Can you work these out from the model? Positions are in its coordinate system, mm. Face numbers are marked on the shaded views. Round coordinates to 2 decimals unless told otherwise and drop trailing zeros. Order: outer loops, then holes, each group sorted by start corner. A loop starts at its lowest first (then second) coordinate and runs counter-clockwise, first axis right, second up. Notation, with made-up numbers: (27.5, 4.25) -> (53.5, 4.25) arc R25 cw to (53.5, 34.25) -> close; hole circle Ø6 at (6.5, 34). An arc over 180 degrees is marked (long way). Use a Markdown table: item, result. Add a question column.
Q1. If we section it at B-B on x = 147: List the corners of the cut face in (y, z) for me, plus the area to 4 significant figures.
Q2. I'm going to push flat-ended pins straight in: pin 1 Ø4 at (x, y) = (99, 4) entering from +Z; pin 2 Ø3 at (x, y) = (148, 5) entering from +Z; pin 3 Ø3 at (y, z) = (5, 11.5) entering from -X. Where does each tip first touch, or does it pass through?
Q3. If we section it at C-C on x = 15: List the corners of the cut face in (y, z) for me.
Q4. If we section it at A-A on x = 88.5: List the corners of the cut face in (y, z) for me, plus the area to 3 significant figures.
Q5. We'd pull the mould along X, two halves only. Please class the marked faces 1 and 2: +X half, -X half, draft (parallel to the pull), parting line (faces both ways), or undercut.
Q6. I need wall thicknesses on line 1 along Y through (x, z) = (15, 1.55); line 2 along Z through (x, y) = (125, 3); line 3 along Z through (x, y) = (150, 6.25). Which ranges of each line are inside material? Lowest first, please. Write a range as [from, to].
Autodesk Inventor part; units mm, degrees
ref_plane "YZ Plane" through (0, 0, 0) normal (1, 0, 0) x (0, 1, 0)
ref_plane "XZ Plane" through (0, 0, 0) normal (0, 1, 0) x (-1, 0, 0)
ref_plane "XY Plane" through (0, 0, 0) normal (0, 0, 1) x (1, 0, 0)
sketch "Sketch1" plane through (0, 0, 0) normal (0, 0, 1) x (1, 0, 0)
  line L0 (0, 0) -> (164.5, 0)
  line L1 (164.5, 0) -> (164.5, 9)
  line L2 (164.5, 9) -> (0, 9)
  line L3 (0, 9) -> (0, 0)
  circle A0 centre (57, 4) radius 1.6
  circle A1 centre (99, 4) radius 1.6
  circle A2 centre (159.5, 4) radius 1.6
  circle A3 centre (147, 4) radius 1.6
  circle A4 centre (15, 4) radius 1.6
  circle A5 centre (7, 4) radius 1.6
  dimension "d1" = 9
  dimension "d2" = 90
  dimension "d4" = 3.2
  dimension "d6" = 3.2
  dimension "d7" = 3.2
  dimension "d8" = 42
  dimension "d9" = 60.5
  dimension "d26" = 3.2
  dimension "d27" = 48
  dimension "d28" = 3.2
  dimension "d29" = 42
  dimension "d32" = 15
  dimension "d33" = 5
  dimension "d61" = 3.2
  dimension "d62" = 8
  dimension "d63" = 12.5
  dimension "d108" = 4
  dimension "d109" = 4
  dimension "d110" = 4
  dimension "d111" = 4
  dimension "d112" = 4
  dimension "d113" = 4
ref_plane "Work Plane2" through (0, 0, 0) normal (0, -1, 0) x (1, 0, 0)
sketch "Sketch2" plane through (0, 0, 0) normal (0, -1, 0) x (1, 0, 0)
  circle A0 centre (52, 10) radius 1.6
  circle A1 centre (125, 10) radius 1.6
  circle A2 centre (88.5, 10) radius 1.6
  point P0 (0, 0)
  point P1 (52, 0)
  dimension "d13" = 3.2
  dimension "d15" = 3.2
  dimension "d17" = 3.2
  dimension "d18" = 36.5
  dimension "d64" = 52
  dimension "d65" = 36.5
  dimension "d114" = 10
  dimension "d115" = 73
ref_plane "Work Plane1" through (0, 0, 11) normal (0, 0, 1) x (1, 0, 0)
extrude "klocek" add sketch "Sketch1" along normal blind 13
ref_plane "Work Plane3" through (0, 0, 0) normal (0, -1, 0) x (1, 0, 0)
extrude "prowadzenie osi" cut sketch "Sketch2" against normal up to next
ref_plane "Work Plane4" through (0, 0, 0) normal (0, -1, 0) x (1, 0, 0)
sketch "Sketch7" plane through (0, 0, 0) normal (0, -1, 0) x (1, 0, 0)
  line L0 (0, 13) -> (0, 1)
  line L1 (0, 13) -> (164.5, 13)
  line L2 (0, 13) -> (40, 13)
  line L3 (40, 13) -> (0, 1)
  point P0 (0, -1.8333)
  dimension "d86" = 12
  dimension "d87" = 40
sketch "Sketch8" plane through (0, 0, 0) normal (0, -1, 0) x (1, 0, 0)
  line L0 (164.5, 0) -> (164.5, 13)
  line L1 (164.5, 13) -> (164.5, 1)
  line L2 (164.5, 13) -> (0, 13)
  line L3 (164.5, 13) -> (134.5, 13)
  line L4 (134.5, 13) -> (164.5, 1)
  point P0 (0, 0)
  point P1 (40.8333, 11)
  dimension "d80" = 12
  dimension "d81" = 30
extrude "przedni skos" cut sketch "Sketch7" against normal up to next
extrude "tylni skos" cut sketch "Sketch8" against normal up to next
ref_plane "Work Plane7" through (0, 0, 11) normal (0, 0, 1) x (1, 0, 0)
sketch "Sketch5" plane through (0, 0, 13) normal (0, 0, 1) x (1, 0, 0)
  circle A0 centre (99, 4) radius 1.6
  line L0 (95.5936, 4) -> (97.2968, 6.95)
  line L1 (97.2968, 6.95) -> (100.7032, 6.95)
  line L2 (100.7032, 6.95) -> (102.4064, 4)
  line L3 (102.4064, 4) -> (100.7032, 1.05)
  line L4 (100.7032, 1.05) -> (97.2968, 1.05)
  line L5 (97.2968, 1.05) -> (95.5936, 4)
  circle A1 centre (57, 4) radius 1.6
  line L6 (60.4064, 4) -> (58.7032, 1.05)
  line L7 (58.7032, 1.05) -> (55.2968, 1.05)
  line L8 (55.2968, 1.05) -> (53.5936, 4)
  line L9 (53.5936, 4) -> (55.2968, 6.95)
  line L10 (55.2968, 6.95) -> (58.7032, 6.95)
  line L11 (58.7032, 6.95) -> (60.4064, 4)
  point P0 (119.5, 5)
  dimension "d98" = 5.9
  dimension "d100" = 5.9
extrude "hex insert middle" cut sketch "Sketch5" against normal blind 3
ref_plane "Work Plane6" through (0, 0, 11) normal (0, 0, 1) x (1, 0, 0)
sketch "Sketch9" plane through (0, 0, 11) normal (0, 0, 1) x (1, 0, 0)
  circle A0 centre (147, 4) radius 1.6
  line L0 (150.4064, 4) -> (148.7032, 1.05)
  line L1 (148.7032, 1.05) -> (145.2968, 1.05)
  line L2 (145.2968, 1.05) -> (143.5936, 4)
  line L3 (143.5936, 4) -> (145.2968, 6.95)
  line L4 (145.2968, 6.95) -> (148.7032, 6.95)
  line L5 (148.7032, 6.95) -> (150.4064, 4)
  point P0 (0, 0)
  point P1 (153, 5)
  dimension "d99" = 5.9
extrude "hex insert rear 1" cut sketch "Sketch9" against normal blind 7.5
ref_plane "Work Plane5" through (0, 0, 11) normal (0, 0, 1) x (1, 0, 0)
sketch "Sketch10" plane through (0, 0, 11) normal (0, 0, 1) x (1, 0, 0)
  circle A0 centre (159.5, 4) radius 1.6
  line L0 (162.45, 5.7032) -> (162.45, 2.2968)
  line L1 (162.45, 2.2968) -> (159.5, 0.5936)
  line L2 (159.5, 0.5936) -> (156.55, 2.2968)
  line L3 (156.55, 2.2968) -> (156.55, 5.7032)
  line L4 (156.55, 5.7032) -> (159.5, 7.4064)
  line L5 (159.5, 7.4064) -> (162.45, 5.7032)
  line L6 (164.5, 0) -> (134.5, 0)
  point P0 (0, 0)
  dimension "d118" = 5.9
extrude "hex insert rear 2" cut sketch "Sketch10" against normal up to next contours A0 | L0 L1 L2 L3 L4 L5
sketch "Sketch13" plane through (0, 0, 11) normal (0, 0, 1) x (1, 0, 0)
  circle A0 centre (7, 4) radius 1.6
  line L0 (10.4064, 4) -> (8.7032, 1.05)
  line L1 (8.7032, 1.05) -> (5.2968, 1.05)
  line L2 (5.2968, 1.05) -> (3.5936, 4)
  line L3 (3.5936, 4) -> (5.2968, 6.95)
  line L4 (5.2968, 6.95) -> (8.7032, 6.95)
  line L5 (8.7032, 6.95) -> (10.4064, 4)
  dimension "d123" = 5.9
extrude "hex insert front 1" cut sketch "Sketch13" against normal through all
sketch "Sketch16" plane through (0, 0, 11) normal (0, 0, 1) x (1, 0, 0)
  circle A0 centre (15, 4) radius 1.6
  line L0 (18.4064, 4) -> (16.7032, 1.05)
  line L1 (16.7032, 1.05) -> (13.2968, 1.05)
  line L2 (13.2968, 1.05) -> (11.5936, 4)
  line L3 (11.5936, 4) -> (13.2968, 6.95)
  line L4 (13.2968, 6.95) -> (16.7032, 6.95)
  line L5 (16.7032, 6.95) -> (18.4064, 4)
  point P0 (0, 0)
  dimension "d93" = 5.9
extrude "hex insert front 2" cut sketch "Sketch16" against normal blind 9
sketch "Sketch17" plane through (0, 0, 0) normal (0, 0, -1) x (-1, 0, 0)
  line L0 (-164.5, 9) -> (0, 9)
  line L1 (0, 0) -> (-2, 0)
  line L2 (-2, 0) -> (-2, 9)
  line L3 (-2, 9) -> (0, 9)
  line L4 (0, 9) -> (0, 0)
  dimension "d122" = 2
extrude "ciecie przod" cut sketch "Sketch17" against normal up to next
sketch "Sketch18" plane through (40, 0, 13) normal (0, -1, 0) x (1, 0, 0)
  line L0 (9.5, 0) -> (9.5, -4)
  line L1 (9.5, -4) -> (-15.5, -4)
  line L2 (-15.5, -4) -> (-15.5, 0)
  line L3 (-15.5, 0) -> (9.5, 0)
  line L4 (94.5, 0) -> (0, 0)
  circle A0 centre (12, -3) radius 1.6
  line L5 (-40, -13) -> (124.5, -13)
  point P0 (-35, -11)
  dimension "d102" = 4
  dimension "d103" = 25
  dimension "d104" = 2.5
extrude "sensor linii" cut sketch "Sketch18" against normal blind 7.3 contours L0 L1 L2 L3
properties part number "wheel_support_v5_narrow_with_line_sensor_all_holes_2mm_higher"
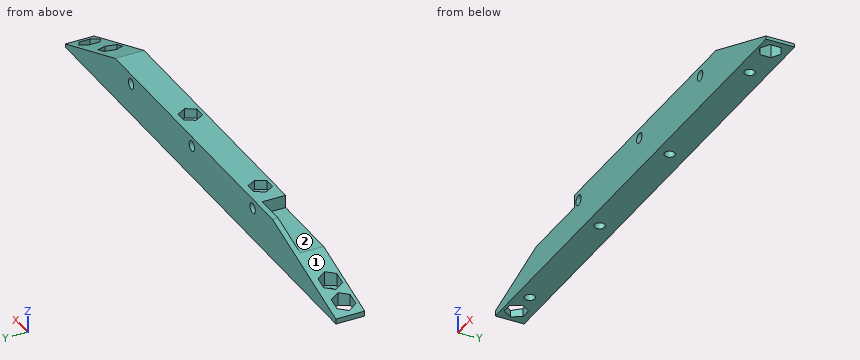
Answer below:
| question | item | result |
|---|---|---|
| 1 | outline | (0, 0) -> (2.4, 0) -> (2.4, 3.5) -> (1.05, 3.5) -> (1.05, 8) -> (0, 8) -> close; (5.6, 0) -> (9, 0) -> (9, 8) -> (6.95, 8) -> (6.95, 3.5) -> (5.6, 3.5) -> close |
| 1 | area | 34.25 mm² |
| 2 | pin 1 | z = 10 |
| 2 | pin 2 | z = 3.5 |
| 2 | pin 3 | x = 49.5 |
| 3 | outline | (0, 0) -> (2.4, 0) -> (2.4, 2) -> (1.05, 2) -> (1.05, 5.5) -> (0, 5.5) -> close; (5.6, 0) -> (9, 0) -> (9, 5.5) -> (6.95, 5.5) -> (6.95, 2) -> (5.6, 2) -> close |
| 4 | outline | (0, 0) -> (9, 0) -> (9, 8.4) -> (0, 8.4) -> close; (0, 11.6) -> (9, 11.6) -> (9, 13) -> (0, 13) -> close |
| 4 | area | 88.2 mm² |
| 5 | face 1 | -X half |
| 5 | face 2 | draft |
| 6 | line 1 | [0, 2.4], [5.6, 9] |
| 6 | line 2 | [0, 8.4], [11.6, 13] |
| 6 | line 3 | [0, 6.8] |
